Work out the finished part from the listing and answer in its coordinate system (mm). A direction names the side the tool comes from. Give positions to 0.01 mm unless a question says otherwise; leave off trailing zeros. Order: outer loops, then holes, each group sorted by start corner. A loop starts at its lowest first (then second) coordinate and runs counter-clockwise, first axis right, second up.
```python
from build123d import *
from build123d.topology import SkipClean

# Parameters (mm, degrees)
SKETCH_1_R                     = 34
EXTRUDE_2_DEPTH                = 5
EXTRUDE_3_DEPTH                = 8
EXTRUDE_START                  = -3
SKETCH_3_R                     = 46.25
SKETCH_3_R_2                   = 34
EXTRUDE_4_DEPTH                = 3
EXTRUDE_5_DEPTH                = 27.3
EXTRUDE_5_DEPTH_BACK           = 3
SKETCH_4_R                     = 51.25
SKETCH_4_R_2                   = 46.25
SKETCH_5_R                     = 58
SKETCH_5_R_2                   = 51.25
EXTRUDE_6_DEPTH                = 5
HOLE_WIZARD_M4_1_D             = 3.3
HOLE_WIZARD_M4_1_CSINK_D       = 4.05
HOLE_WIZARD_M4_1_CSINK_ANGLE   = 90
PATTERN_CIRCULAR_1_COUNT       = 6
HOLE_WIZARD_M3_5_1_D           = 2.9
HOLE_WIZARD_M3_5_1_CSINK_D     = 3.55
HOLE_WIZARD_M3_5_1_CSINK_ANGLE = 90
PATTERN_CIRCULAR_2_COUNT       = 8
SKETCH_10_R                    = 58
CUT_EXTRUDE_1_DEPTH            = 27.3


with BuildPart() as part:
    # Sketch 1 → Extrude 2 (new body)
    with BuildSketch(Plane(origin=(0, 0, 0), x_dir=(1, 0, 0), z_dir=(0, 1, 0))):
        with Locations(Location((0, 0, 0), (0, 0, 270))):
            Circle(SKETCH_1_R)
    extrude(amount=EXTRUDE_2_DEPTH)

    # Sketch 2 → Extrude 3 (add)
    with SkipClean():  # the faces are left unmerged after this step: merging them gives an invalid solid
        with BuildSketch(Plane(origin=(0, 5, 0), x_dir=(1, 0, 0), z_dir=(0, 1, 0))):
            with BuildLine():
                Line((-34, 0), (-29, 0))
                ThreePointArc((-29, 0), (-25.11473671, 14.5), (-14.5, 25.11473671))
                Line((-14.5, 25.11473671), (-17, 29.444863729))
                ThreePointArc((-17, 29.444863729), (-29.444863729, 17), (-34, 0))
            make_face()
            with BuildLine():
                Line((29, 0), (34, 0))
                ThreePointArc((34, 0), (29.444863729, -17), (17, -29.444863729))
                Line((17, -29.444863729), (14.5, -25.11473671))
                ThreePointArc((14.5, -25.11473671), (25.11473671, -14.5), (29, 0))
            make_face()
        extrude(amount=EXTRUDE_3_DEPTH)

    # Sketch 3 → Extrude 4 (add)
    with SkipClean():  # the faces are left unmerged after this step: merging them gives an invalid solid
        with BuildSketch(Plane(origin=(0, 13, 0), x_dir=(1, 0, 0), z_dir=(0, 1, 0)).offset(EXTRUDE_START)):
            with Locations(Location((0, 0, 0), (0, 0, 270))):
                Circle(SKETCH_3_R)
            with Locations(Location((0, 0, 0), (0, 0, 120))):
                Circle(SKETCH_3_R_2, mode=Mode.SUBTRACT)
        extrude(amount=EXTRUDE_4_DEPTH)

    # Sketch 4 → Extrude 5 (add, two sides: drawn at the far end of the back side and taken through both)
    with SkipClean():  # the faces are left unmerged after this step: merging them gives an invalid solid
        with BuildSketch(Plane(origin=(0, 13, 0), x_dir=(1, 0, 0), z_dir=(0, 1, 0)).offset(-EXTRUDE_5_DEPTH_BACK)):
            with Locations(Location((0, 0, 0), (0, 0, 270))):
                Circle(SKETCH_4_R)
            with Locations(Location((0, 0, 0), (0, 0, 270))):
                Circle(SKETCH_4_R_2, mode=Mode.SUBTRACT)
        extrude(amount=EXTRUDE_5_DEPTH + EXTRUDE_5_DEPTH_BACK)

    # Sketch 5 → Extrude 6 (add)
    with SkipClean():  # the faces are left unmerged after this step: merging them gives an invalid solid
        with BuildSketch(Plane(origin=(0, 40.3, 0), x_dir=(1, 0, 0), z_dir=(0, 1, 0))):
            with Locations(Location((0, 0, 0), (0, 0, 270))):
                Circle(SKETCH_5_R)
            with Locations(Location((0, 0, 0), (0, 0, 270))):
                Circle(SKETCH_5_R_2, mode=Mode.SUBTRACT)
        extrude(amount=-EXTRUDE_6_DEPTH)

    # Hole Wizard M4 _1 (through all)
    with Locations(Plane.XZ):
        with Locations((8.625, -14.938938215)):
            hole_wizard_m4_1 = CounterSinkHole(HOLE_WIZARD_M4_1_D / 2, HOLE_WIZARD_M4_1_CSINK_D / 2, counter_sink_angle=HOLE_WIZARD_M4_1_CSINK_ANGLE)

    # Pattern Circular 1: Hole Wizard M4 _1 ×6 about axis
    with SkipClean():  # the faces are left unmerged after this step: merging them gives an invalid solid
        pattern_circular_1_axis = Axis((0, 0, 0), (0, 1, 0))
        for i in range(1, PATTERN_CIRCULAR_1_COUNT):
            add(hole_wizard_m4_1.rotate(pattern_circular_1_axis, i * 360 / PATTERN_CIRCULAR_1_COUNT), mode=Mode.SUBTRACT)

    # Hole Wizard M3.5 _1 (through all)
    with Locations(Plane.XZ.offset(-10)):
        with Locations((36.806079661, 21.25)):
            hole_wizard_m3_5_1 = CounterSinkHole(HOLE_WIZARD_M3_5_1_D / 2, HOLE_WIZARD_M3_5_1_CSINK_D / 2, counter_sink_angle=HOLE_WIZARD_M3_5_1_CSINK_ANGLE)

    # Pattern Circular 2: Hole Wizard M3.5 _1 ×8 about axis
    with SkipClean():  # the faces are left unmerged after this step: merging them gives an invalid solid
        pattern_circular_2_axis = Axis((0, 0, 0), (0, 1, 0))
        for i in range(1, PATTERN_CIRCULAR_2_COUNT):
            add(hole_wizard_m3_5_1.rotate(pattern_circular_2_axis, i * 360 / PATTERN_CIRCULAR_2_COUNT), mode=Mode.SUBTRACT)

    # Sketch 10 → Cut-Extrude 1 (cut)
    with SkipClean():  # the faces are left unmerged after this step: merging them gives an invalid solid
        with BuildSketch(Plane(origin=(0, 40.3, 0), x_dir=(1, 0, 0), z_dir=(0, 1, 0))):
            Circle(SKETCH_10_R)
        extrude(amount=-CUT_EXTRUDE_1_DEPTH, mode=Mode.SUBTRACT)


solid = part.part
```
1. Which of the six approach directions +Z, -Z, +X, -X, +Y, -Y give full straight-line access (tool end or side, diameter ignored) to faces 3 (the face through (-15.6, 2.72, 0.07)), 4 (the face through (-15.732, 8.944, -27.249)), 5 (the face through (-11, 10, 33))?
Findings below:
face 3: +Y, -Y
face 4: +Y
face 5: -Y
2. Given P1, Ø4, axis at x = 18.5, y = 1.5, coming from the -Z side; P2, Ø5.5, axis at x = -31.5, y = 7.5, coming from the +Z side; P3, Ø3, axis at x = 38.5, z = -25.5, coming from the -Y side, each flat-ended and moving along its own axis, determine where each tip first touches the part or whether it passes through.
Findings below:
P1: stops at z = -29.73
P2: stops at z = 41.29
P3: stops at y = 10
3. The part is cut by section A-A (x = 0). Write down the section's boundary in (y, z).
Findings below:
outline: (0, -34) - (5, -34) - (5, 34) - (0, 34) - close; (10, -51.25) - (13, -51.25) - (13, -34) - (10, -34) - close; (10, 34) - (13, 34) - (13, 51.25) - (10, 51.25) - close
4. The part is cut by section D-D (z = -21.25). Write down the section's boundary in (x, y) (3 decimals), then the cut area to 3 significant figures.
Findings below:
outline: (-46.637, 10) - (-38.581, 10) - (-38.256, 10.325) - (-38.256, 13) - (-46.637, 13) - close; (-35.356, 10.325) - (-35.031, 10) - (-26.541, 10) - (-26.541, 0) - (26.541, 0) - (26.541, 5) - (-19.734, 5) - (-19.734, 13) - (-35.356, 13) - close; (26.541, 10) - (46.637, 10) - (46.637, 13) - (26.541, 13) - close
area: 432 mm2
5. The mould has two halves that part along Z. Classify faces 1 (the face through (0, 5, 0)), 2 (the face through (-17.43, 11.479, 29.192)): pulls with the +Z half, pulls with the -Z half, needs draft (parallel to the pull), parting line crosses it, or undercut.
Findings below:
face 1: needs draft
face 2: undercut
6. The part is cut by section B-B (z = -7.5). Write down the section's boundary in (x, y).
Findings below:
outline: (-50.7, 10) - (-33.16, 10) - (-33.16, 0) - (33.16, 0) - (33.16, 5) - (-28.01, 5) - (-28.01, 13) - (-50.7, 13) - close; (33.16, 10) - (50.7, 10) - (50.7, 13) - (33.16, 13) - close
7. The part is cut by section C-C (y = 2.5). Write down the section's boundary in (x, z) (3 decimals), then the cut area to 3 significant figures.
Findings below:
outline: circle Ø68 at (0, 0); hole circle Ø3.3 at (-17.25, 0); hole circle Ø3.3 at (-8.625, -14.939); hole circle Ø3.3 at (-8.625, 14.939); hole circle Ø3.3 at (8.625, -14.939); hole circle Ø3.3 at (8.625, 14.939); hole circle Ø3.3 at (17.25, 0)
area: 3,580 mm2
8. Straight lines are drawn through the part: probe 1 along X at (y, z) = (11.5, 21.25); probe 2 along Z at (x, y) = (-21.25, 10.95); probe 3 along Y at (x, z) = (-23.5, -45.5). For each, find the intervals that lie inside material, in ascending order.
Findings below:
probe 1: x = -46.64 to -26.54, 19.73 to 35.36, 38.26 to 46.64
probe 2: z = -46.64 to -19.73, 26.54 to 35.36, 38.26 to 46.64
probe 3: y = 10 to 13
